Read the model definition and answer for the solid it produces. Units are mm, in the model's axes. Coordinates: 2 decimals unless noted, no trailing zeros. Loops run counter-clockwise (first coordinate to the right, second up) from the corner with the lowest first, then second, coordinate; pieces in that order, holes last.
from build123d import *

# Parameters (mm, degrees)
SKETCH1_R           = 2.5
BOSS_EXTRUDE1_DEPTH = 5


with BuildPart() as part:
    # Sketch1 → Boss-Extrude1 (new body)
    with BuildSketch(Plane(origin=(0, 0, 0), x_dir=(1, 0, 0), z_dir=(0, 1, 0))):
        with BuildLine():
            Line((20, -25), (-20, -25))
            ThreePointArc((-20, -25), (-23.535533906, -23.535533906), (-25, -20))
            Line((-25, -20), (-25, 20))
            ThreePointArc((-25, 20), (-23.535533906, 23.535533906), (-20, 25))
            Line((-20, 25), (20, 25))
            ThreePointArc((20, 25), (23.535533906, 23.535533906), (25, 20))
            Line((25, 20), (25, -20))
            ThreePointArc((25, -20), (23.535533906, -23.535533906), (20, -25))
        make_face()
        with Locations((-20, 20)):
            Circle(SKETCH1_R, mode=Mode.SUBTRACT)
        with Locations((-10, 20)):
            Circle(SKETCH1_R, mode=Mode.SUBTRACT)
        with Locations((0, 20)):
            Circle(SKETCH1_R, mode=Mode.SUBTRACT)
        with Locations((10, 20)):
            Circle(SKETCH1_R, mode=Mode.SUBTRACT)
        with Locations((20, 20)):
            Circle(SKETCH1_R, mode=Mode.SUBTRACT)
        with Locations((-10, 10)):
            Circle(SKETCH1_R, mode=Mode.SUBTRACT)
        with Locations((0, 10)):
            Circle(SKETCH1_R, mode=Mode.SUBTRACT)
        with Locations((10, 10)):
            Circle(SKETCH1_R, mode=Mode.SUBTRACT)
        with Locations((20, 10)):
            Circle(SKETCH1_R, mode=Mode.SUBTRACT)
        with Locations((-10, 0)):
            Circle(SKETCH1_R, mode=Mode.SUBTRACT)
        Circle(SKETCH1_R, mode=Mode.SUBTRACT)
        with Locations((10, 0)):
            Circle(SKETCH1_R, mode=Mode.SUBTRACT)
        with Locations((20, 0)):
            Circle(SKETCH1_R, mode=Mode.SUBTRACT)
        with Locations((-10, -10)):
            Circle(SKETCH1_R, mode=Mode.SUBTRACT)
        with Locations((0, -10)):
            Circle(SKETCH1_R, mode=Mode.SUBTRACT)
        with Locations((10, -10)):
            Circle(SKETCH1_R, mode=Mode.SUBTRACT)
        with Locations((20, -10)):
            Circle(SKETCH1_R, mode=Mode.SUBTRACT)
        with Locations((-10, -20)):
            Circle(SKETCH1_R, mode=Mode.SUBTRACT)
        with Locations((0, -20)):
            Circle(SKETCH1_R, mode=Mode.SUBTRACT)
        with Locations((10, -20)):
            Circle(SKETCH1_R, mode=Mode.SUBTRACT)
        with Locations((20, -20)):
            Circle(SKETCH1_R, mode=Mode.SUBTRACT)
        with Locations((-20, 10)):
            Circle(SKETCH1_R, mode=Mode.SUBTRACT)
        with Locations((-20, 0)):
            Circle(SKETCH1_R, mode=Mode.SUBTRACT)
        with Locations((-20, -10)):
            Circle(SKETCH1_R, mode=Mode.SUBTRACT)
        with Locations((-20, -20)):
            Circle(SKETCH1_R, mode=Mode.SUBTRACT)
    extrude(amount=BOSS_EXTRUDE1_DEPTH)


solid = part.part
Q1. A flat-ended cylindrical pin translates along its axis: pin 1 Ø3 at (x, z) = (-20, 0) entering from +Y. Find the tip coordinate at first contact, or state that the pin passes through.
Findings below:
pin 1: passes through
Q2. Determine the mould class of faces 1 (the face through (0, 2, 25)), 2 (the face through (-10.33, 2.46, -22.48)), 3 (the face through (23, 2, -24)), 4 (the face through (-23, 2, 24)) for opening direction X: +X half, -X half, draft (parallel to the pull), parting line (faces both ways), or undercut.
Findings below:
face 1: draft
face 2: undercut
face 3: +X half
face 4: -X half
Q3. A cutting plane is placed at C-C (y = 3.25). Count the separate pieces of the cut face and the enclosed holes in it, then the cut area to 3 significant figures.
Findings below:
separate pieces: 1
enclosed holes: 25
area: 1,990 mm2
Q4. A cutting plane is placed at A-A (z = -10). Give the vertices of the cut face in (x, y).
Findings below:
outline: (-25, 0) - (-22.5, 0) - (-22.5, 5) - (-25, 5) - close; (-17.5, 0) - (-12.5, 0) - (-12.5, 5) - (-17.5, 5) - close; (-7.5, 0) - (-2.5, 0) - (-2.5, 5) - (-7.5, 5) - close; (2.5, 0) - (7.5, 0) - (7.5, 5) - (2.5, 5) - close; (12.5, 0) - (17.5, 0) - (17.5, 5) - (12.5, 5) - close; (22.5, 0) - (25, 0) - (25, 5) - (22.5, 5) - close
Q5. A cutting plane is placed at B-B (x = -10). Give the vertices of the cut face in (y, z), then the cut area to 3 significant figures.
Findings below:
outline: (0, -25) - (5, -25) - (5, -22.5) - (0, -22.5) - close; (0, -17.5) - (5, -17.5) - (5, -12.5) - (0, -12.5) - close; (0, -7.5) - (5, -7.5) - (5, -2.5) - (0, -2.5) - close; (0, 2.5) - (5, 2.5) - (5, 7.5) - (0, 7.5) - close; (0, 12.5) - (5, 12.5) - (5, 17.5) - (0, 17.5) - close; (0, 22.5) - (5, 22.5) - (5, 25) - (0, 25) - close
area: 125 mm2
Q6. Straight lines are drawn through the part: probe 1 along X at (y, z) = (2.2, -20); probe 2 along Z at (x, y) = (-18, 1.8). For each, find the intervals that lie inside material, in ascending order.
Findings below:
probe 1: x = -25 to -22.5, -17.5 to -12.5, -7.5 to -2.5, 2.5 to 7.5, 12.5 to 17.5, 22.5 to 25
probe 2: z = -25 to -21.5, -18.5 to -11.5, -8.5 to -1.5, 1.5 to 8.5, 11.5 to 18.5, 21.5 to 25
